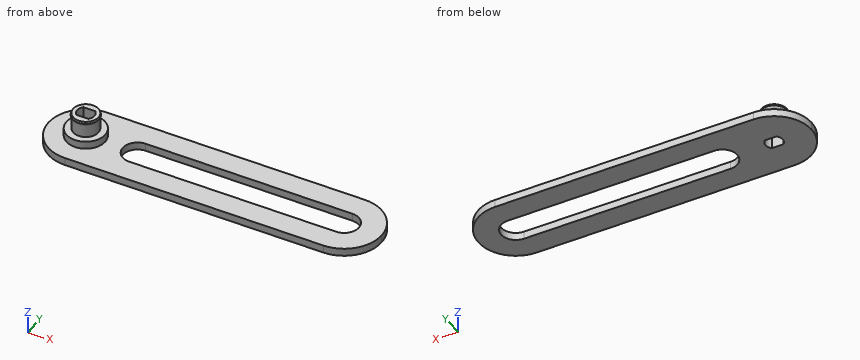
from build123d import *

# Parameters (mm, degrees)
F4_R      = 7.5
F4_R_2    = 5.5
F5_DEPTH  = 3
F6_DEPTH  = 5
F7_R      = 9.5
F7_R_2    = 7.5
F7_R_3    = 4.9
F8_DEPTH  = 3
F9_DEPTH  = 6
F10_DEPTH = 12.5


with BuildPart() as f5:
    # F4 (on Top) → F5 (new body)
    with BuildSketch(Plane.XY):
        with BuildLine():
            Line((100, 14.5), (0, 14.5))
            ThreePointArc((0, 14.5), (-10.2530483272, 10.2530483272), (-14.5, 0))
            ThreePointArc((-14.5, 0), (-10.2530483272, -10.2530483272), (0, -14.5))
            Line((0, -14.5), (100, -14.5))
            ThreePointArc((100, -14.5), (110.2530483272, -10.2530483272), (114.5, 0))
            ThreePointArc((114.5, 0), (110.2530483272, 10.2530483272), (100, 14.5))
        make_face()
        Circle(F4_R, mode=Mode.SUBTRACT)
        with BuildLine():
            ThreePointArc((20, -5.7), (14.3, 0), (20, 5.7))
            Line((20, 5.7), (100, 5.7))
            ThreePointArc((100, 5.7), (105.7, 0), (100, -5.7))
            Line((100, -5.7), (20, -5.7))
        make_face(mode=Mode.SUBTRACT)
        Circle(F4_R)
        Circle(F4_R_2, mode=Mode.SUBTRACT)
    extrude(amount=F5_DEPTH)

    # F4 (on Top) → F6 (join)
    with BuildSketch(Plane.XY):
        Circle(F4_R)
        Circle(F4_R_2, mode=Mode.SUBTRACT)
    extrude(amount=F6_DEPTH)



with BuildPart() as f8:
    # F7 (on Top) → F8 (new body)
    with BuildSketch(Plane.XY):
        Circle(F7_R)
        Circle(F7_R_2, mode=Mode.SUBTRACT)
        Circle(F7_R_2)
        Circle(F7_R_3, mode=Mode.SUBTRACT)
        Circle(F7_R_3)
        with BuildLine():
            ThreePointArc((-2.2847319318, -2.45), (-3.35, 0), (-2.2847319318, 2.45))
            Line((-2.2847319318, 2.45), (2.2847319318, 2.45))
            ThreePointArc((2.2847319318, 2.45), (3.35, 0), (2.2847319318, -2.45))
            Line((2.2847319318, -2.45), (-2.2847319318, -2.45))
        make_face(mode=Mode.SUBTRACT)
    extrude(amount=F8_DEPTH)


with BuildPart() as f5_1:
    add(f5.part)

    add(f8.part)  # F9 merges F8
    # F7 (on Top) → F9 (join)
    with BuildSketch(Plane.XY):
        Circle(F7_R_2)
        Circle(F7_R_3, mode=Mode.SUBTRACT)
        Circle(F7_R_3)
        with BuildLine():
            ThreePointArc((-2.2847319318, -2.45), (-3.35, 0), (-2.2847319318, 2.45))
            Line((-2.2847319318, 2.45), (2.2847319318, 2.45))
            ThreePointArc((2.2847319318, 2.45), (3.35, 0), (2.2847319318, -2.45))
            Line((2.2847319318, -2.45), (-2.2847319318, -2.45))
        make_face(mode=Mode.SUBTRACT)
    extrude(amount=F9_DEPTH)

    # F7 (on Top) → F10 (join)
    with BuildSketch(Plane.XY):
        Circle(F7_R_3)
        with BuildLine():
            ThreePointArc((-2.2847319318, -2.45), (-3.35, 0), (-2.2847319318, 2.45))
            Line((-2.2847319318, 2.45), (2.2847319318, 2.45))
            ThreePointArc((2.2847319318, 2.45), (3.35, 0), (2.2847319318, -2.45))
            Line((2.2847319318, -2.45), (-2.2847319318, -2.45))
        make_face(mode=Mode.SUBTRACT)
    extrude(amount=F10_DEPTH)

    # F11 (on Front) → F12 (revolve)
    with BuildSketch(Plane.XZ):
        Polygon((5.15, 11.75), (4.9, 12.5), (4.9, 11), align=None)
    revolve(axis=Axis((0, 0, 8.631802164), (0, 0, 1)))


solid = f5_1.part
The model under review builds one solid part; all positions refer to its coordinate system, in mm. Give positions to 0.01 mm unless a question says otherwise; leave off trailing zeros. Loops run counter-clockwise (first coordinate to the right, second up) from the corner with the lowest first, then second, coordinate; pieces in that order, holes last. Notation, with made-up numbers: (25, -10) -> (32, -10) arc R31 cw to (32, 23) -> close; hole circle Ø4 at (-10.75, 62). An arc over 180 degrees is marked (long way). Put each result on its own line as item: value. Start each with the question number.
1. Clearance check with flat-ended pins moving along their axes: P1, Ø6, axis at y = 7.5, z = 9.5, coming from the -X side; P2, Ø3.5, axis at x = 1, z = 9.5, coming from the -Y side; P3, Ø3.5, axis at x = 0.5, z = 8.5, coming from the +Y side. State where each tip first meets the part, or that it passes through.
2. We need section A-A on x = 87.5. State the section outline as (y, z) points, then the cut area to 3 significant figures.
3. Wall thickness on probe 1 along X at (y, z) = (0.25, 1.25); probe 2 along Z at (x, y) = (37, 8.5); probe 3 along X at (y, z) = (-3, 2.5): over which ranges is each line inside the solid? List them lowest first.
4. We need section C-C on y = -12. State the section outline as (x, z) points.
5. We need section B-B on z = 8.5. State the section outline as (x, y) points.
Determined:
1. P1: x = -1.94
1. P2: y = -4.93
1. P3: y = 4.9
2. outline: (-14.5, 0) -> (-5.7, 0) -> (-5.7, 3) -> (-14.5, 3) -> close; (5.7, 0) -> (14.5, 0) -> (14.5, 3) -> (5.7, 3) -> close
2. area: 52.8 mm^2
3. probe 1: -14.5 to -3.34, 3.34 to 14.31, 105.69 to 114.5
3. probe 2: 0 to 3
3. probe 3: -14.19 to 15.15, 104.85 to 114.19
4. outline: (-8.14, 0) -> (108.14, 0) -> (108.14, 3) -> (-8.14, 3) -> close
5. outline: circle Ø9.8 at (0, 0); hole (-2.28, -2.45) -> (2.28, -2.45) arc R3.35 ccw to (2.28, 2.45) -> (-2.28, 2.45) arc R3.35 ccw to start
